Read the model definition and answer for the solid it produces. Units are mm, in the model's axes. Face numbers are marked on the shaded views. Give positions to 0.01 mm unless a question says otherwise; leave off trailing zeros. Write each loop counter-clockwise with the first axis right and the second up, starting at its lowest first coordinate (ties: lowest second). Pieces come first, ordered by that corner, then holes. Notation, with made-up numbers: (82.5, -10.5) -> (96.5, -10.5) arc R19 ccw to (96.5, 21.5) -> close; hole circle Ø6 at (-29, 41). An arc over 180 degrees is marked (long way). Put each result on its own line as item: value. Start each with the question number.
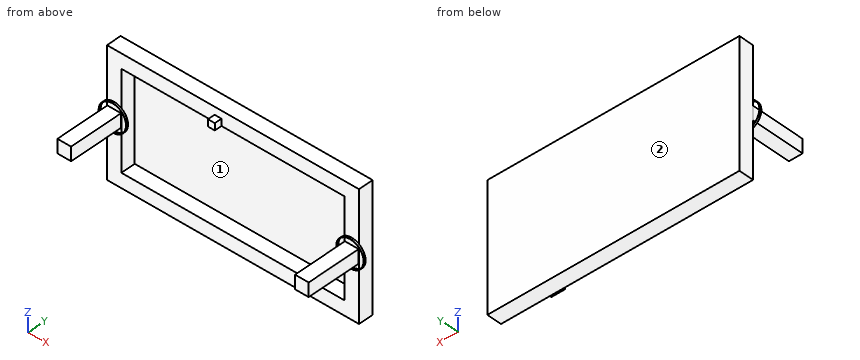
from build123d import *

# Parameters (mm, degrees)
SKETCH1_W           = 700
SKETCH1_H           = 350
SKETCH1_W_2         = 620
SKETCH1_H_2         = 270
BOSS_EXTRUDE1_DEPTH = 40
SKETCH2_W           = 700
SKETCH2_H           = 350
BOSS_EXTRUDE2_DEPTH = 1
SKETCH3_W           = 38
SKETCH3_H           = 38
BOSS_EXTRUDE3_DEPTH = 150
SKETCH4_W           = 19
SKETCH4_H           = 19
BOSS_EXTRUDE4_DEPTH = 20
SKETCH5_R           = 38.5
SKETCH5_R_2         = 37.5
BOSS_EXTRUDE5_DEPTH = 5


with BuildPart() as part:
    # Sketch1 → Boss-Extrude1 (new body)
    with BuildSketch(Plane(origin=(0, 0, 0), x_dir=(1, 0, 0), z_dir=(0, 1, 0))):
        Rectangle(SKETCH1_W, SKETCH1_H)
        Rectangle(SKETCH1_W_2, SKETCH1_H_2, mode=Mode.SUBTRACT)
    extrude(amount=BOSS_EXTRUDE1_DEPTH)

    # Sketch2 → Boss-Extrude2 (add)
    with BuildSketch(Plane(origin=(0, 40, 0), x_dir=(1, 0, 0), z_dir=(0, 1, 0))):
        Rectangle(SKETCH2_W, SKETCH2_H)
    extrude(amount=BOSS_EXTRUDE2_DEPTH)

    # Sketch3 → Boss-Extrude3 (add)
    with BuildSketch(Plane.XZ):
        with Locations((-330, 0)):
            Rectangle(SKETCH3_W, SKETCH3_H)
        with Locations((330, 0)):
            Rectangle(SKETCH3_W, SKETCH3_H)
    extrude(amount=BOSS_EXTRUDE3_DEPTH)

    # Sketch4 → Boss-Extrude4 (add)
    with BuildSketch(Plane.XZ):
        with Locations((-41.5, 144.5)):
            Rectangle(SKETCH4_W, SKETCH4_H)
    extrude(amount=BOSS_EXTRUDE4_DEPTH)

    # Sketch5 → Boss-Extrude5 (add)
    with BuildSketch(Plane.XZ):
        with Locations((-330, 0)):
            Circle(SKETCH5_R)
        with Locations((-330, 0)):
            Circle(SKETCH5_R_2, mode=Mode.SUBTRACT)
        with Locations((330, 0)):
            Circle(SKETCH5_R)
        with Locations((330, 0)):
            Circle(SKETCH5_R_2, mode=Mode.SUBTRACT)
    extrude(amount=BOSS_EXTRUDE5_DEPTH)


solid = part.part
1) A cutting plane is placed at D-D on y = 24. Give the vertices of the cut face in (x, z), and give its area (3 significant figures).
2) A cutting plane is placed at B-B on z = 0. State how many separate pieces and enclosed holes the cut face has, and give its area (3 significant figures).
3) A cutting plane is placed at C-C on x = 330. Give the vertices of the cut face in (y, z), and give its area (3 significant figures).
4) A cutting plane is placed at A-A on y = -120. Give the vertices of the cut face in (x, z).
5) Each of these flat-tipped pins is pushed along its axis until it touches: pin 1 Ø5.5 at (y, z) = (-10.5, 141) entering from -X; pin 2 Ø12 at (y, z) = (22, 41) entering from +X; pin 3 Ø19 at (x, y) = (-327, -84) entering from +Z. Where does it stop, or does it pass through?
6) For a pull along X with two mould halves and no side action, classify the marked faces 1 and 2 as pulls with the +X half, pulls with the -X half, needs draft (parallel to the pull), parting line crosses it, or undercut.
7) Straight lines are drawn through the part: line 1 (Z direction, x = -330, y = -1.5); line 2 (X direction, y = -2, z = 0); line 3 (Z direction, x = -175, y = 14.5). For each, find the intervals that lie inside material, in ascending order. Write a range as [from, to].
Results found:
1. outline: (-350, -175) -> (350, -175) -> (350, 175) -> (-350, 175) -> close; hole (-310, -135) -> (310, -135) -> (310, 135) -> (-310, 135) -> close
1. area: 77,600 mm²
2. separate pieces: 5
2. enclosed holes: 0
2. area: 15,300 mm²
3. outline: (-150, -19) -> (0, -19) -> (0, -37.5) -> (-5, -37.5) -> (-5, -38.5) -> (0, -38.5) -> (0, -175) -> (41, -175) -> (41, 175) -> (0, 175) -> (0, 38.5) -> (-5, 38.5) -> (-5, 37.5) -> (0, 37.5) -> (0, 19) -> (-150, 19) -> close
3. area: 20,100 mm²
4. outline: (-349, -19) -> (-311, -19) -> (-311, 19) -> (-349, 19) -> close; (311, -19) -> (349, -19) -> (349, 19) -> (311, 19) -> close
5. pin 1: stops at x = -51
5. pin 2: stops at x = 350
5. pin 3: stops at z = 19
6. face 1: undercut
6. face 2: needs draft
7. line 1: z = [-38.5, -37.5], [-19, 19], [37.5, 38.5]
7. line 2: x = [-368.5, -367.5], [-349, -311], [-292.5, -291.5], [291.5, 292.5], [311, 349], [367.5, 368.5]
7. line 3: z = [-175, -135], [135, 175]
